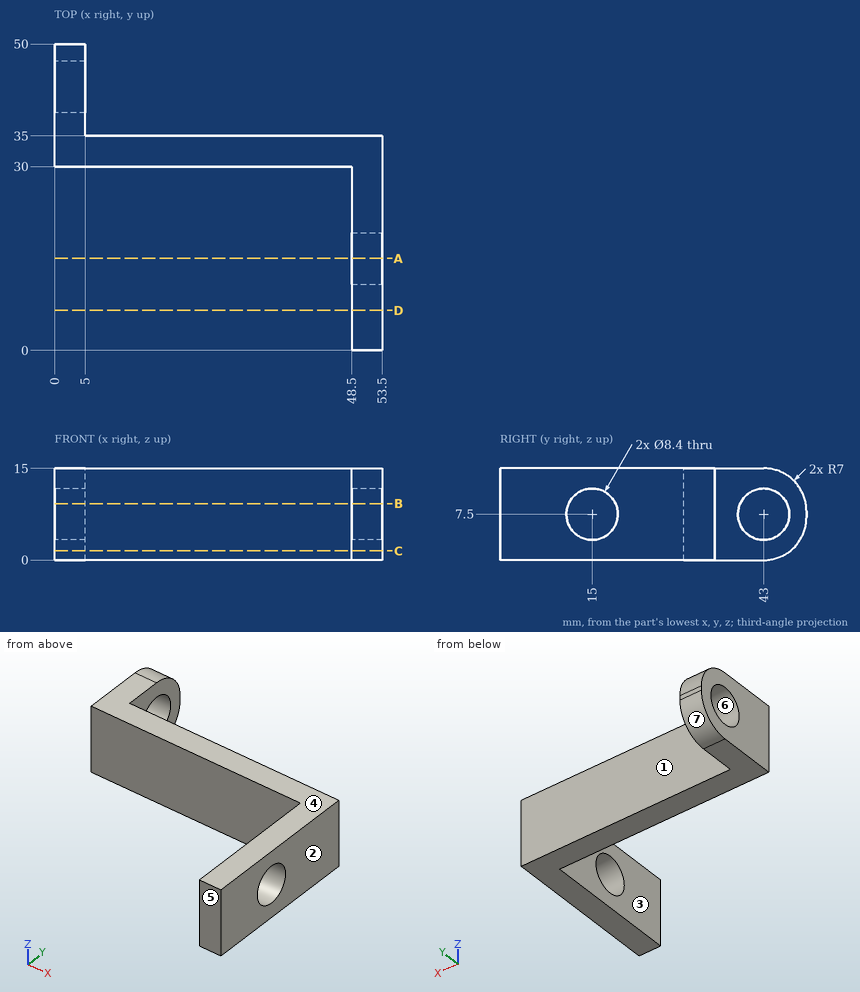
For this review, use the dimensioned drawing (mm, ordinates from the lowest corner) and the shaded views. A direction names the side the tool comes from. Round coordinates to 2 decimals unless told otherwise and drop trailing zeros. Write each loop counter-clockwise with the first axis right and the second up, starting at its lowest first coordinate (ties: lowest second). Pieces come first, ordered by that corner, then holes. Notation, with made-up numbers: (-13.75, 10.25) -> (11.25, 10.25) arc R6 cw to (11.25, 21.25) -> close; hole circle Ø6 at (72, 22.25). An arc over 180 degrees is marked (long way). Answer in a Markdown table with one row per item.
Q1. Take a section at B-B, the plane z = 9.25. State the section outline as (x, y) points.
The answers:
| item | result |
|---|---|
| outline | (0, 30) -> (48.5, 30) -> (48.5, 18.82) -> (53.5, 18.82) -> (53.5, 35) -> (5, 35) -> (5, 39.18) -> (0, 39.18) -> close; (0, 46.82) -> (5, 46.82) -> (5, 49.89) -> (0, 49.89) -> close; (48.5, 0) -> (53.5, 0) -> (53.5, 11.18) -> (48.5, 11.18) -> close |
Q2. Take a section at C-C, the plane z = 1.5. State the section outline as (x, y) points, then the cut area to 3 significant figures.
The answers:
| item | result |
|---|---|
| outline | (0, 30) -> (48.5, 30) -> (48.5, 0) -> (53.5, 0) -> (53.5, 35) -> (5, 35) -> (5, 47.33) -> (0, 47.33) -> close |
| area | 479 mm² |
Q3. Clearance check with flat-ended pins moving along their axes: pin 1 Ø4 at (x, z) = (16.5, 3.5) entering from +Y; pin 2 Ø3 at (x, z) = (43.5, 6) entering from -Y; pin 3 Ø4.5 at (y, z) = (9, 5) entering from -X. State where each tip first meets the part, or that it passes through.
The answers:
| item | result |
|---|---|
| pin 1 | y = 35 |
| pin 2 | y = 30 |
| pin 3 | x = 48.5 |
Q4. For the marked faces 1, 2 and 3, list the 3-axis set-ups (+Z, -Z, +X, -X, +Y, -Y) from which the entire face can be reached by the end or side of a thin tool; tool diameter is ignored.
The answers:
| item | result |
|---|---|
| face 1 | +Z, -Z, +X, +Y |
| face 2 | +Z, -Z, +X, +Y, -Y |
| face 3 | +Z, -Z, -X, -Y |
Q5. To check wall thickness, follow L1, parallel to Y at x = 1.8, z = 7.5; L2, parallel to Y at x = 50.25, z = 7.5; L3, parallel to Z at x = 52, y = 15. State the ranges of each line that lie inside material, in increasing order. Write a range as [from, to].
The answers:
| item | result |
|---|---|
| L1 | [30, 38.8], [47.2, 50] |
| L2 | [0, 10.8], [19.2, 35] |
| L3 | [0, 3.3], [11.7, 15] |
Q6. Take a section at D-D, the plane y = 6.5. State the section outline as (x, z) points, then the cut area to 3 significant figures.
The answers:
| item | result |
|---|---|
| outline | (48.5, 0) -> (53.5, 0) -> (53.5, 15) -> (48.5, 15) -> close |
| area | 75.0 mm² |
Q7. Draft analysis for pull direction Z (two halves, no side actions). For the marked faces 4, 5, 6 and 7, state which applies: +Z half, -Z half, draft (parallel to the pull), parting line (faces both ways), or undercut.
The answers:
| item | result |
|---|---|
| face 4 | +Z half |
| face 5 | draft |
| face 6 | undercut |
| face 7 | -Z half |
Q8. Take a section at A-A, the plane y = 15. State the section outline as (x, z) points.
The answers:
| item | result |
|---|---|
| outline | (48.5, 0) -> (53.5, 0) -> (53.5, 3.3) -> (48.5, 3.3) -> close; (48.5, 11.7) -> (53.5, 11.7) -> (53.5, 15) -> (48.5, 15) -> close |
